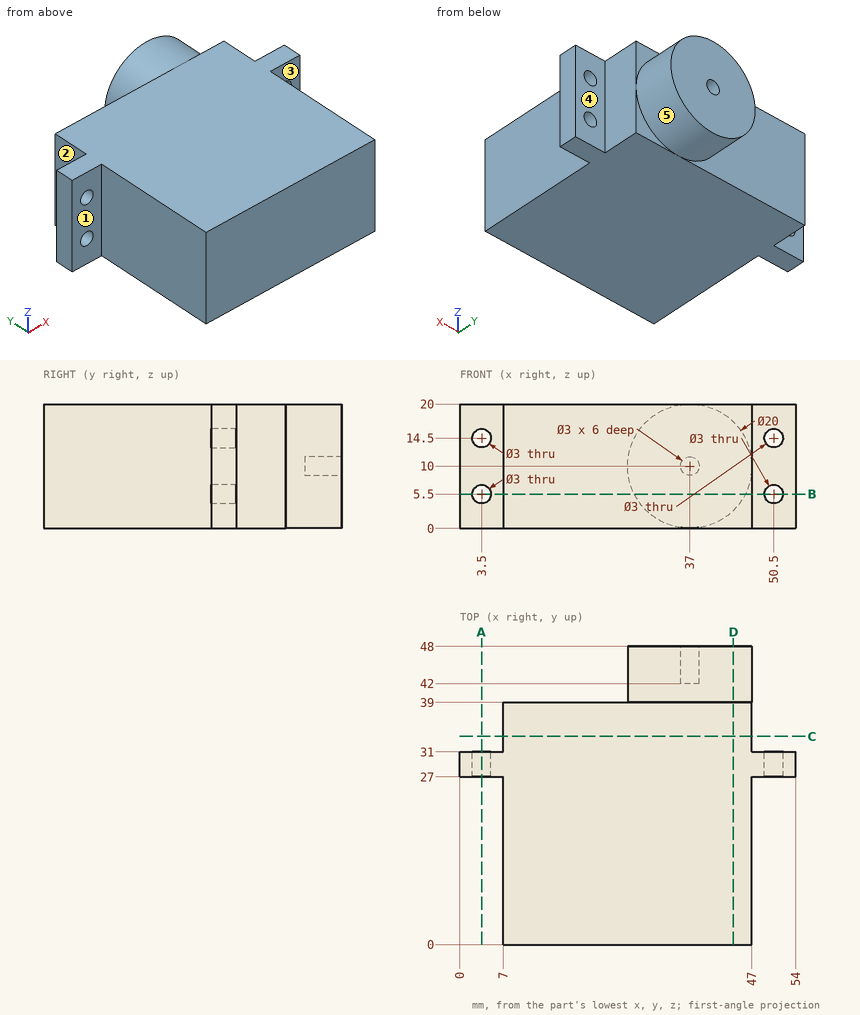
Input: dimensioned drawing with shaded views. Units: mm. Origin: part minimum x, y, z. A direction names the side the tool comes from. Coordinates: 2 decimals unless noted, no trailing zeros. Order: outer loops, then holes, each group sorted by start corner. A loop starts at its lowest first (then second) coordinate and runs counter-clockwise, first axis right, second up. Notation, with made-up numbers: M 28,89.5 L 58,89.5 A11 cw 58,97.5 Z; hole C 36,5 d1. An arc over 180 degrees is marked long. Write each question's results on one line, items separated by ' | '. Start each with the question number.
Item 1: First-contact query: pin 1 Ø2 at (y, z) = (24.5, 3.5) entering from +X; pin 2 Ø2 at (x, z) = (2.5, 10) entering from +Y; pin 3 Ø2 at (x, z) = (4, 8) entering from -Y. Flat tips, straight axial feed; report the tip coordinate or a pass-through.
Item 2: Cut plane D-D (x = 44). Return loops of the section in (y, z).
Item 3: Set-up query: the marked faces 1, 2, 3, 4 and 5. Return all of +Z, -Z, +X, -X, +Y, -Y with unobstructed straight access to the full face (end or side cutting, diameter ignored); none if empty.
Item 4: Cut plane C-C (y = 33.5). Return loops of the section in (x, z).
Item 5: Cut plane B-B (z = 5.5). Return loops of the section in (x, y), and give its area (3 significant figures).
Item 6: Cut plane A-A (x = 3.5). Return loops of the section in (y, z), and give its area (3 significant figures).
Item 7: Line query: probe 1 along X at (y, z) = (28.5, 14.5); probe 2 along X at (y, z) = (32, 1.5); probe 3 along Y at (x, z) = (13, 7.25). Output: solid intervals per line, ascending.
Checked values:
1) pin 1: stops at x = 47 | pin 2: stops at y = 31 | pin 3: stops at y = 27
2) outline: M 0,0 L 39,0 L 39,2.86 L 48,2.86 L 48,17.14 L 39,17.14 L 39,20 L 0,20 Z
3) face 1: +Z, -Z, -X, -Y | face 2: +Z, -Z, -X, +Y | face 3: +Z, -Z, +X, -Y | face 4: +Z, -Z, +X, +Y | face 5: +Y
4) outline: M 7,0 L 47,0 L 47,20 L 7,20 Z
5) outline: M 0,27 L 2,27 L 2,31 L 0,31 Z; M 5,27 L 7,27 L 7,0 L 47,0 L 47,27 L 49,27 L 49,31 L 47,31 L 47,39 L 45.93,39 L 45.93,48 L 28.07,48 L 28.07,39 L 7,39 L 7,31 L 5,31 Z; M 52,27 L 54,27 L 54,31 L 52,31 Z | area: 1,750 mm2
6) outline: M 27,0 L 31,0 L 31,4 L 27,4 Z; M 27,7 L 31,7 L 31,13 L 27,13 Z; M 27,16 L 31,16 L 31,20 L 27,20 Z | area: 56.0 mm2
7) probe 1: x = 0 to 2, 5 to 49, 52 to 54 | probe 2: x = 7 to 47 | probe 3: y = 0 to 39
